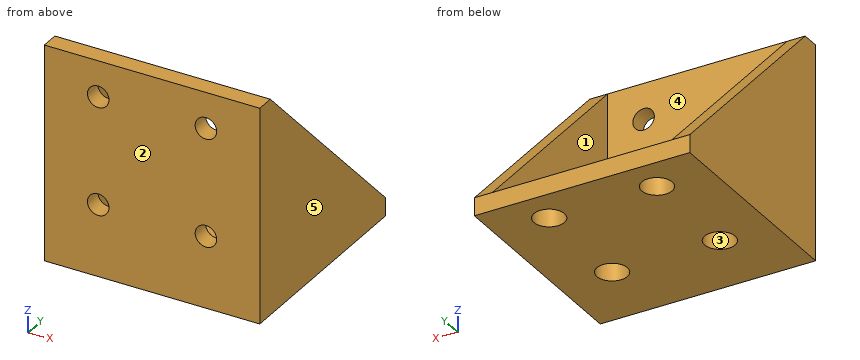
```python
from build123d import *

# Parameters (mm, degrees)
F1_DEPTH  = 60
F3_DEPTH  = 5
F6_DEPTH  = 5
F7_R      = 3
F8_DEPTH  = 5.001
F9_R      = 4.25
F10_DEPTH = 5.001


with BuildPart() as f1:
    # F0 (on Right) → F1 (new body)
    with BuildSketch(Plane.YZ):
        Polygon((5, 60), (0, 60), (0, 0), (60, 0), (60, 5), (5, 5), align=None)
    extrude(amount=F1_DEPTH)

    # F2 (on Right) → F3 (join)
    with BuildSketch(Plane.YZ):
        Polygon((60, 5), (5, 60), (5, 5), align=None)
    extrude(amount=F3_DEPTH)

    # F5 (on offset) → F6 (join)
    with BuildSketch(Plane.YZ.offset(60)):
        Polygon((60, 5), (5, 60), (5, 5), align=None)
    extrude(amount=-F6_DEPTH)

    # F7 (on face) → F8 (cut, through all)
    with BuildSketch(Plane(origin=(0, 5, 0), x_dir=(-1, 0, 0), z_dir=(0, 1, 0))):
        with Locations((-15, 50)):
            Circle(F7_R)
        with Locations((-45, 50)):
            Circle(F7_R)
        with Locations((-15, 20)):
            Circle(F7_R)
        with Locations((-45, 20)):
            Circle(F7_R)
    extrude(amount=-F8_DEPTH, mode=Mode.SUBTRACT)

    # F9 (on face) → F10 (cut, through all)
    with BuildSketch(Plane.XY.offset(5)):
        with Locations((45, 50)):
            Circle(F9_R)
        with Locations((15, 50)):
            Circle(F9_R)
        with Locations((15, 20)):
            Circle(F9_R)
        with Locations((45, 20)):
            Circle(F9_R)
    extrude(amount=-F10_DEPTH, mode=Mode.SUBTRACT)


solid = f1.part
```
Work out the finished part from the listing and answer in its coordinate system (mm). Face numbers are marked on the shaded views. A direction names the side the tool comes from. Give positions to 0.01 mm unless a question says otherwise; leave off trailing zeros. Order: outer loops, then holes, each group sorted by start corner. A loop starts at its lowest first (then second) coordinate and runs counter-clockwise, first axis right, second up. Notation, with made-up numbers: M 48,87.5 L 102,87.5 A19 ccw 102,113.5 Z; hole C 74,66.25 d9. An arc over 180 degrees is marked long. Return JSON: item names as keys, results as strings.
1) Straight lines are drawn through the part: line 1 along Y through (x, z) = (45, 3.1); line 2 along Z through (x, y) = (45, 1.25); line 3 along X through (y, z) = (8.5, 54.5). For each, find the intervals that lie inside material, in ascending order. Write a range as [from, to].
Resolved:
{"line 1": "[0, 15.75], [24.25, 45.75], [54.25, 60]", "line 2": "[0, 17], [23, 47], [53, 60]", "line 3": "[0, 5], [55, 60]"}
2) Section C-C, the plane z = 50 is taken. Write down the section's boundary in (x, y), plus the area to 3 significant figures.
Resolved:
{"outline": "M 0,0 L 12,0 L 12,5 L 5,5 L 5,15 L 0,15 Z; M 18,0 L 42,0 L 42,5 L 18,5 Z; M 48,0 L 60,0 L 60,15 L 55,15 L 55,5 L 48,5 Z", "area": "340 mm^2"}
3) A tool of negligible diameter and unlimited length cuts with its end or side. For the marked faces 4 and 5, from which of +Z, -Z, +X, -X, +Y, -Y can it reach the whole face along a straight path? Write none if from no direction.
Resolved:
{"face 4": "+Z, +Y", "face 5": "+Z, -Z, +X, +Y, -Y"}
4) Each of these flat-tipped pins is pushed along its axis until it touches: pin 1 (12 mm diameter, centred on x = 17.5, z = 18, fed in from +Y); pin 2 (15 mm diameter, centred on x = 29, y = 27.5, fed in from +Z). Where does it stop, or does it pass through?
Resolved:
{"pin 1": "y = 5", "pin 2": "z = 5"}
5) Section B-B, the plane y = 50 is taken. Write down the section's boundary in (x, z), plus the area to 3 significant figures.
Resolved:
{"outline": "M 0,0 L 10.75,0 L 10.75,5 L 5,5 L 5,15 L 0,15 Z; M 19.25,0 L 40.75,0 L 40.75,5 L 19.25,5 Z; M 49.25,0 L 60,0 L 60,15 L 55,15 L 55,5 L 49.25,5 Z", "area": "315 mm^2"}
6) Section D-D, the plane y = 8.5 is taken. Write down the section's boundary in (x, z), plus the area to 3 significant figures.
Resolved:
{"outline": "M 0,0 L 60,0 L 60,56.5 L 55,56.5 L 55,5 L 5,5 L 5,56.5 L 0,56.5 Z", "area": "815 mm^2"}
7) Section A-A, the plane x = 15 is taken. Write down the section's boundary in (y, z), plus the area to 3 significant figures.
Resolved:
{"outline": "M 0,0 L 15.75,0 L 15.75,5 L 5,5 L 5,17 L 0,17 Z; M 0,23 L 5,23 L 5,47 L 0,47 Z; M 0,53 L 5,53 L 5,60 L 0,60 Z; M 24.25,0 L 45.75,0 L 45.75,5 L 24.25,5 Z; M 54.25,0 L 60,0 L 60,5 L 54.25,5 Z", "area": "430 mm^2"}
8) For a pull along Y with two mould halves and no side action, classify the marked faces 1, 2 and 3 as +Y half, -Y half, draft (parallel to the pull), parting line (faces both ways), or undercut.
Resolved:
{"face 1": "draft", "face 2": "-Y half", "face 3": "undercut"}
